Design review of the part built by this model. Coordinates are the model's own, in mm. Face numbers are marked on the shaded views. Round coordinates to 2 decimals unless told otherwise and drop trailing zeros. Order: outer loops, then holes, each group sorted by start corner. A loop starts at its lowest first (then second) coordinate and runs counter-clockwise, first axis right, second up. Notation, with made-up numbers: (-7.5, 26.25) - (38.5, 26.25) arc R26 cw to (38.5, 48.25) - close; hole circle Ø10 at (-8, 44). An arc over 180 degrees is marked (long way). Write item = value, one per line.
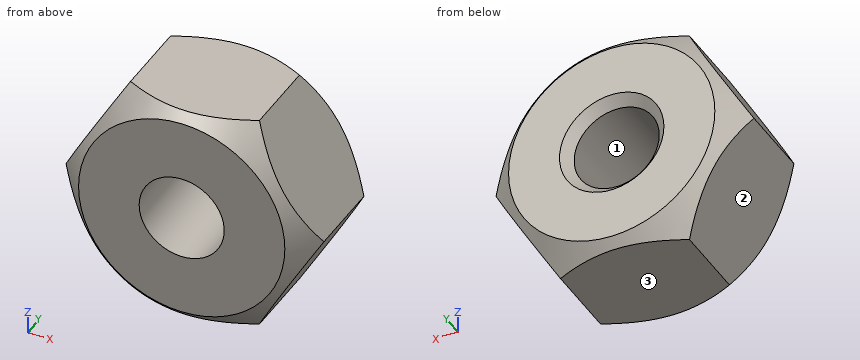
from build123d import *

# Parameters (mm, degrees)
BOSS_EXTRUDE1_DEPTH             = 2.5
M4X0_7_TAPPED_HOLE1_D           = 3.3
M4X0_7_TAPPED_HOLE1_DEPTH       = 9.108579979
M4X0_7_TAPPED_HOLE1_CSINK_D     = 4.05
M4X0_7_TAPPED_HOLE1_CSINK_ANGLE = 90
M4X0_7_TAPPED_HOLE1_TIP         = 0.991420021


with BuildPart() as part:
    # Sketch1 → Boss-Extrude1 (new, symmetric)
    with BuildSketch(Plane(origin=(0, 0, 0), x_dir=(1, 0, 0), z_dir=(0, 1, 0))):
        Polygon((2.5, -4.330127019), (5, 0), (2.5, 4.330127019), (-2.5, 4.330127019), (-5, 0), (-2.5, -4.330127019), align=None)
    extrude(amount=BOSS_EXTRUDE1_DEPTH, both=True)

    # Sketch2 → Cut-Revolve1 (revolve, cut)
    with BuildSketch(Plane.XY, mode=Mode.PRIVATE) as cut_revolve1_sk:
        Polygon((4, 2.5), (5, 1.5), (5, 2.5), align=None)
    cut_revolve1 = revolve(cut_revolve1_sk.sketch.rotate(Axis((0, 0, 0), (0, 1, 0)), 90), axis=Axis((0, 0, 0), (0, 1, 0)), mode=Mode.SUBTRACT)

    # Mirror1: Cut-Revolve1 across plane
    add(cut_revolve1.mirror(Plane.ZX), mode=Mode.SUBTRACT)

    # M4x0.7 Tapped Hole1
    with Locations(Plane(origin=(0, 2.5, 0), x_dir=(1, 0, 0), z_dir=(0, 1, 0))):
        with Locations((0, 0)):
            CounterSinkHole(M4X0_7_TAPPED_HOLE1_D / 2, M4X0_7_TAPPED_HOLE1_CSINK_D / 2, depth=M4X0_7_TAPPED_HOLE1_DEPTH, counter_sink_angle=M4X0_7_TAPPED_HOLE1_CSINK_ANGLE)
            with Locations((0, 0, -(M4X0_7_TAPPED_HOLE1_DEPTH + M4X0_7_TAPPED_HOLE1_TIP / 2))):  # 118° drill point
                Cone(0, M4X0_7_TAPPED_HOLE1_D / 2, M4X0_7_TAPPED_HOLE1_TIP, mode=Mode.SUBTRACT)


solid = part.part
Item 1: Insertion check: P1, Ø3, axis at y = 1, z = -1, coming from the -X side. The pin has a flat end and moves straight along its axis. Give the tip position at first contact, or say it passes through.
Data:
P1 = -5
Item 2: Take a section at A-A, the plane y = 0.2. State the section outline as (x, z) points, and give its area (3 significant figures).
Data:
outline = (-5, 0) - (-2.5, -4.33) - (2.5, -4.33) - (5, 0) - (2.5, 4.33) - (-2.5, 4.33) - close; hole circle Ø3.3 at (0, 0)
area = 56.4 mm2
Item 3: Take a section at C-C, the plane y = -1.65. State the section outline as (x, z) points.
Data:
outline = (-4.84, -0.27) - (-2.66, -4.06) arc R4.85 ccw to (-2.18, -4.33) - (2.18, -4.33) arc R4.85 ccw to (2.66, -4.06) - (4.84, -0.27) arc R4.85 ccw to (4.84, 0.27) - (2.66, 4.06) arc R4.85 ccw to (2.18, 4.33) - (-2.18, 4.33) arc R4.85 ccw to (-2.66, 4.06) - (-4.84, 0.27) arc R4.85 ccw to start; hole circle Ø3.3 at (0, 0)
Item 4: The part is to be moulded in two halves that separate along X. For the marked faces 1, 2 and 3, say which applies: +X half, -X half, draft (parallel to the pull), parting line (faces both ways), or undercut.
Data:
face_1 = undercut
face_2 = -X half
face_3 = draft
Item 5: For line 1 along Z through (x, y) = (-1, -0.85); line 2 along X through (y, z) = (-0.35, 0.5); line 3 along X through (y, z) = (-1.9, 0.5), list the stretches that pass through material, from the lowest coordinate up. Write a range as [from, to].
Data:
line_1 = [-4.33, -1.31], [1.31, 4.33]
line_2 = [-4.71, -1.57], [1.57, 4.71]
line_3 = [-4.57, -1.57], [1.57, 4.57]
Item 6: Take a section at B-B, the plane x = 0. State the section outline as (y, z) points (3 decimals), and give its area (3 significant figures).
Data:
outline = (-2.5, -4) - (-2.17, -4.33) - (2.17, -4.33) - (2.5, -4) - (2.5, -2.025) - (2.125, -1.65) - (-2.5, -1.65) - close; (-2.5, 1.65) - (2.125, 1.65) - (2.5, 2.025) - (2.5, 4) - (2.17, 4.33) - (-2.17, 4.33) - (-2.5, 4) - close
area = 26.4 mm2
